The figure shows three views and two pictorial views of one solid part (mm, origin at its lowest corner). Answer the questions. A direction names the side the tool comes from. Coordinates: 2 decimals unless noted, no trailing zeros. Order: outer loops, then holes, each group sorted by start corner. A loop starts at its lowest first (then second) coordinate and runs counter-clockwise, first axis right, second up. Notation, with made-up numbers: M 55.25,67 L 89.25,67 A26 ccw 89.25,97 Z; hole C 60,89 d9. An arc over 180 degrees is marked long. Answer in a Markdown table with one row per item. Add a question column.
Item 1: The part is cut by section B-B (y = 78.5). Write down the section's boundary in (x, z), then the cut area to 3 significant figures.
Item 2: The part is cut by section C-C (z = 46). Write down the section's boundary in (x, y).
Item 3: The part is cut by section D-D (x = 70.5). Write down the section's boundary in (y, z) (1 decimal).
Item 4: Consider line 1 (X direction, y = 56, z = 9); line 2 (Y direction, x = 110, z = 13); line 3 (Y direction, x = 132.5, z = 72) (1 decimal). Determine where each line is inside the solid, lowest interval first. Write a range as from..to.
Item 5: The part is cut by section A-A (z = 70). Write down the section's boundary in (x, y), then the cut area to 3 significant figures.
Item 6: A flat-ended cylindrical pin translates along its axis: pin 1 Ø12 at (x, z) = (119.5, 66) entering from -Y. Find the tip coordinate at first contact, or state that the pin passes through.
Item 7: Which of the six approach directions +Z, -Z, +X, -X, +Y, -Y give full straight-line access (tool end or side, diameter ignored) to the marked faces 4 and 5?
Item 8: The mould has two halves that part along Z. Classify the marked faces 1, 2 and 3: released by +Z, released by -Z, zero draft, split by the parting line, or undercut.
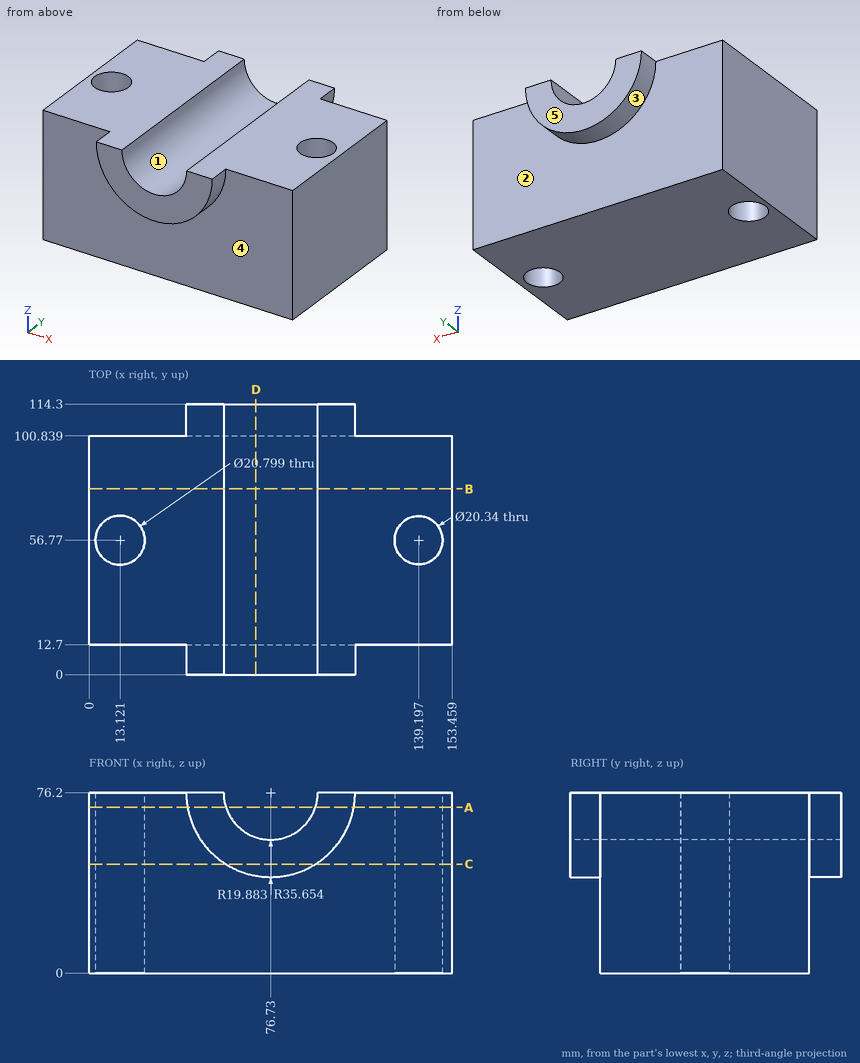
Reply:
| question | item | result |
|---|---|---|
| 1 | outline | M 0,0 L 153.46,0 L 153.46,76.2 L 96.61,76.2 A19.88 cw 56.85,76.2 L 0,76.2 Z |
| 1 | area | 11,100 mm2 |
| 2 | outline | M 0,12.7 L 57.78,12.7 L 57.78,0 L 95.68,0 L 95.68,12.7 L 153.46,12.7 L 153.46,100.84 L 95.68,100.84 L 95.68,114.3 L 57.78,114.3 L 57.78,100.84 L 0,100.84 Z; hole C 13.12,56.77 d20.8; hole C 139.2,56.77 d20.34 |
| 3 | outline | M 0,41.1 L 12.7,41.1 L 12.7,0 L 100.8,0 L 100.8,41.1 L 114.3,41.1 L 114.3,57.3 L 0,57.3 Z |
| 4 | line 1 | x = 0..2.75, 23.49..129.06, 149.34..153.46 |
| 4 | line 2 | y = 12.7..100.84 |
| 4 | line 3 | y = 12.7..49.1, 64.4..100.8 |
| 5 | outline | M 0,12.7 L 41.62,12.7 L 41.62,0 L 57.84,0 L 57.84,114.3 L 41.62,114.3 L 41.62,100.84 L 0,100.84 Z; M 95.62,0 L 111.84,0 L 111.84,12.7 L 153.46,12.7 L 153.46,100.84 L 111.84,100.84 L 111.84,114.3 L 95.62,114.3 Z; hole C 13.12,56.77 d20.8; hole C 139.2,56.77 d20.34 |
| 5 | area | 10,400 mm2 |
| 6 | pin 1 | stops at y = 12.7 |
| 7 | face 4 | -Z, -Y |
| 7 | face 5 | +Z, -Z, +X, -X, +Y |
| 8 | face 1 | released by +Z |
| 8 | face 2 | zero draft |
| 8 | face 3 | released by -Z |
